Geometry check sheet. Reference: the model listing, model coordinates, mm. A direction names the side the tool comes from. Round coordinates to 2 decimals unless told otherwise and drop trailing zeros. Loops run counter-clockwise (first coordinate to the right, second up) from the corner with the lowest first, then second, coordinate; pieces in that order, holes last. Notation, with made-up numbers: (49.25, 43) -> (83.25, 43) arc R10 cw to (83.25, 55) -> close; hole circle Ø10 at (56, -5.5). An arc over 180 degrees is marked (long way). Use a Markdown table: item, result. Add a question column.
Q1. Sectioned sample at B-B, the plane z = 0. Enter the section's corners in (x, y), then the cut area to 3 significant figures.
Q2. Sectioned sample at D-D, the plane x = 6.25. Enter the section's corners in (y, z) (1 decimal).
Q3. Gauge pin test, flat ends, axial feed: P1, Ø1.5, axis at x = 8, z = 1, coming from the -Y side; P2, Ø1, axis at x = 5.5, z = -3.5, coming from the +Y side. Record the tip position at first contact, or that the pin passes through.
Q4. Sectioned sample at A-A, the plane y = -2. Enter the section's corners in (x, z) (3 decimals), then the cut area to 3 significant figures.
Q5. Release check for a two-part mould opening along Y. For faces 4 (the face through (0, -2, -2)), 5 (the face through (4.383, 0.767, -2.435)), 6 (the face through (6.39, -1.05, -3.33)) record: released by +Y, released by -Y, zero draft, split by the parting line, or undercut.
Q6. Sectioned sample at C-C, the plane y = 0. Enter the section's corners in (x, z) (1 decimal).
Q7. Set-up check for faces 1 (the face through (2.59, -0.9, 3.54)), 2 (the face through (3.81, -4, 0)), 3 (the face through (8.89, -3, 0)): record each of +Z, -Z, +X, -X, +Y, -Y from which the full face is reachable in a straight line by a thin tool's end or side.
Q8. Material ranges on L1, parallel to X at y = -2, z = 3.75; L2, parallel to Y at x = 3, z = 0; L3, parallel to Z at x = 3, y = 0, recorded low to high.
```python
from build123d import *

# Parameters (mm, degrees)
SKETCH1_R               = 4.7625
SKETCH1_R_2             = 2.5527
BOSS_EXTRUDE1_DEPTH     = 8.89
SKETCH2_W               = 5.08
SKETCH2_H               = 1.27
CUT_EXTRUDE1_DEPTH      = 12.153246725
CUT_EXTRUDE1_DEPTH_BACK = 12.153246725
SKETCH7_R               = 0.396875
SKETCH3_W               = 1.1303
SKETCH3_H               = 4.7625


with BuildPart() as part:
    # Sketch1 → Boss-Extrude1 (new body)
    with BuildSketch(Plane(origin=(0, 0, 0), x_dir=(0, 0, -1), z_dir=(1, 0, 0))):
        Circle(SKETCH1_R)
        Circle(SKETCH1_R_2, mode=Mode.SUBTRACT)
    extrude(amount=BOSS_EXTRUDE1_DEPTH)

    # Sketch2 → Cut-Revolve1 (revolve, cut)
    with BuildSketch(Plane.XY, mode=Mode.PRIVATE) as cut_revolve1_sk:
        with Locations((6.35, 4.1275)):
            Rectangle(SKETCH2_W, SKETCH2_H)
    revolve(cut_revolve1_sk.sketch.rotate(Axis((8.89, 0, 0), (-1, 0, 0)), 90), axis=Axis((8.89, 0, 0), (-1, 0, 0)), mode=Mode.SUBTRACT)

    # Sketch7 → Cut-Extrude1 (cut, two sides: drawn at the far end of the back side and taken through both)
    with BuildSketch(Plane(origin=(0, 0, 0), x_dir=(1, 0, 0), z_dir=(0, 1, 0)).offset(-CUT_EXTRUDE1_DEPTH_BACK)):
        with Locations(Location((1.905, 3.81, 0), (0, 0, 270))):
            Circle(SKETCH7_R)
    extrude(amount=CUT_EXTRUDE1_DEPTH + CUT_EXTRUDE1_DEPTH_BACK, mode=Mode.SUBTRACT)

    # Sketch3 → ShaftSetScrew (revolve, cut)
    with BuildSketch(Plane.YZ.offset(1.905)):
        with Locations((0.56515, 2.38125)):
            Rectangle(SKETCH3_W, SKETCH3_H)
    revolve(axis=Axis((1.905, 0, -6.35), (0, 0, 1)), mode=Mode.SUBTRACT)


solid = part.part
```
Values:
| question | item | result |
|---|---|---|
| 1 | outline | (0, -4.76) -> (3.81, -4.76) -> (3.81, -3.49) -> (8.89, -3.49) -> (8.89, -2.55) -> (0, -2.55) -> close; (0, 2.55) -> (8.89, 2.55) -> (8.89, 3.49) -> (3.81, 3.49) -> (3.81, 4.76) -> (0, 4.76) -> close |
| 1 | area | 26.4 mm^2 |
| 2 | outline | circle Ø7 at (0, 0); hole circle Ø5.1 at (0, 0) |
| 3 | P1 | y = -3.48 |
| 3 | P2 | y = 1.79 |
| 4 | outline | (0, -4.322) -> (3.81, -4.322) -> (3.81, -2.863) -> (8.89, -2.863) -> (8.89, -1.586) -> (0, -1.586) -> close; (0, 1.586) -> (8.89, 1.586) -> (8.89, 2.863) -> (3.81, 2.863) -> (3.81, 4.322) -> (0, 4.322) -> close; hole circle Ø0.794 at (1.905, -3.81) |
| 4 | area | 33.3 mm^2 |
| 5 | face 4 | zero draft |
| 5 | face 5 | undercut |
| 5 | face 6 | split by the parting line |
| 6 | outline | (0, -4.8) -> (3.8, -4.8) -> (3.8, -3.5) -> (8.9, -3.5) -> (8.9, -2.6) -> (0, -2.6) -> close; (0, 2.6) -> (0.8, 2.6) -> (0.8, 4.8) -> (0, 4.8) -> close; (3, 2.6) -> (8.9, 2.6) -> (8.9, 3.5) -> (3.8, 3.5) -> (3.8, 4.8) -> (3, 4.8) -> close; hole circle Ø0.8 at (1.9, -3.8) |
| 7 | face 1 | +Z |
| 7 | face 2 | +X |
| 7 | face 3 | +Z, -Z, +X, +Y, -Y |
| 8 | L1 | 0 to 3.81 |
| 8 | L2 | -4.76 to -2.55, 2.55 to 4.76 |
| 8 | L3 | -4.76 to -2.55 |
